Can you work these out from the model? Positions are in its coordinate system, mm. A direction names the side the tool comes from. Round coordinates to 2 decimals unless told otherwise and drop trailing zeros. Loops run counter-clockwise (first coordinate to the right, second up) from the corner with the lowest first, then second, coordinate; pieces in that order, holes last.
(1) Which directions (+Z, -Z, +X, -X, +Y, -Y) give clear straight access to the entire face, cutting with the end or side of a thin tool? Please do faces 1 (the face through (4.606, -3, 3)), 2 (the face through (-1, 150, 3)), 3 (the face through (4.606, 103, 3)).
(2) I want a section at C-C on x = 10.5. Write out the boundary of the cut face in (y, z).
(3) Will these pins go through, and if not, where does the flat tip stop? pin 1 Ø4 at (x, y) = (-20.39, 15) entering from +Z; pin 2 Ø2 at (x, y) = (-0.21, 80) entering from -Z.
(4) Thinking about a two-plate mould opening in X: for faces 4 (the face through (-5.394, -3, 3)), 5 (the face through (-0.48, 38.29, 3.04)), 6 (the face through (-16, 0, 3)), 7 (the face through (19.378, 26.735, 3.042)), which applies, released by +X, released by -X, zero draft, split by the parting line, or undercut?
(5) If I drill on line 1 along X through (y, z) = (65, 1.95); line 2 along Y through (x, z) = (-4, 4.35); line 3 along Y through (x, z) = (-18, 2.9), over which ranges is the centre line in solid material (lowest first)?
(6) I want a section at A-A on y = 40. Write out the boundary of the cut face in (x, z).
(7) I want a section at B-B on z = 4.65. Give the number of separate pieces and of enclosed holes in the cut face, plus the area to 3 significant figures.
from build123d import *

# Parameters (mm, degrees)
ESBO_O1_W                = 50
ESBO_O1_H                = 150
RESSALTO_EXTRUS_O1_DEPTH = 6
ESBO_O2_R                = 1.75
CORTE_EXTRUS_O1_DEPTH    = 6
ESBO_O3_W                = 10
ESBO_O3_H                = 6
RESSALTO_EXTRUS_O2_DEPTH = 6
ESBO_O4_W                = 10
ESBO_O4_H                = 6.295380903
CORTE_EXTRUS_O2_DEPTH    = 6
ESBO_O5_W                = 10
ESBO_O5_H                = 6
CORTE_EXTRUS_O3_DEPTH    = 6


with BuildPart() as part:
    # Esboço1 → Ressalto-extrusão1 (new body)
    with BuildSketch(Plane.XY):
        with Locations((-0.394283087, 75)):
            Rectangle(ESBO_O1_W, ESBO_O1_H)
    extrude(amount=RESSALTO_EXTRUS_O1_DEPTH)

    # Esboço2 → Corte-extrusão1 (cut)
    with BuildSketch(Plane.XY.offset(6)):
        with Locations((-20.394283087, 95)):
            Circle(ESBO_O2_R)
        with Locations((-20.394283087, 85)):
            Circle(ESBO_O2_R)
        with Locations((-20.394283087, 75)):
            Circle(ESBO_O2_R)
        with Locations((-20.394283087, 65)):
            Circle(ESBO_O2_R)
        with Locations((-20.394283087, 55)):
            Circle(ESBO_O2_R)
        with Locations((-20.394283087, 45)):
            Circle(ESBO_O2_R)
        with Locations((-20.394283087, 35)):
            Circle(ESBO_O2_R)
        with Locations((-20.394283087, 25)):
            Circle(ESBO_O2_R)
        with Locations((-20.394283087, 15)):
            Circle(ESBO_O2_R)
        with Locations((-20.394283087, 5)):
            Circle(ESBO_O2_R)
        with Locations((19.605716913, 95)):
            Circle(ESBO_O2_R)
        with Locations((19.605716913, 85)):
            Circle(ESBO_O2_R)
        with Locations((19.793101921, 75)):
            Circle(ESBO_O2_R)
        with Locations((19.793101921, 65)):
            Circle(ESBO_O2_R)
        with Locations((19.793101921, 55)):
            Circle(ESBO_O2_R)
        with Locations((19.605716913, 45)):
            Circle(ESBO_O2_R)
        with Locations((19.605716913, 35)):
            Circle(ESBO_O2_R)
        with Locations((19.605716913, 25)):
            Circle(ESBO_O2_R)
        with Locations((19.605716913, 15)):
            Circle(ESBO_O2_R)
        with Locations((19.605716913, 5)):
            Circle(ESBO_O2_R)
        with Locations((-0.052571078, 20)):
            Circle(ESBO_O2_R)
        with Locations((-0.210284313, 80)):
            Circle(ESBO_O2_R)
        with Locations((-0.105142156, 40)):
            Circle(ESBO_O2_R)
        with Locations((-0.157713235, 60)):
            Circle(ESBO_O2_R)
    extrude(amount=-CORTE_EXTRUS_O1_DEPTH, mode=Mode.SUBTRACT)

    # Esboço3 → Ressalto-extrusão2 (add)
    with BuildSketch(Plane(origin=(0, 0, 0), x_dir=(-1, 0, 0), z_dir=(0, -1, 0))):
        with Locations((0.394283087, -3)):
            Rectangle(ESBO_O3_W, ESBO_O3_H)
    extrude(amount=RESSALTO_EXTRUS_O2_DEPTH)

    # Esboço4 → Corte-extrusão2 (cut)
    with BuildSketch(Plane.XY.offset(6)):
        with Locations((-0.394283087, 103.147690452)):
            Rectangle(ESBO_O4_W, ESBO_O4_H)
    extrude(amount=-CORTE_EXTRUS_O2_DEPTH, mode=Mode.SUBTRACT)

    # Esboço5 → Corte-extrusão3 (cut)
    with BuildSketch(Plane.XY.offset(6)):
        with Locations((-0.394283087, 143.295380903)):
            Rectangle(ESBO_O5_W, ESBO_O5_H)
    extrude(amount=-CORTE_EXTRUS_O3_DEPTH, mode=Mode.SUBTRACT)


solid = part.part
Filled sheet:
1. face 1: +Z, -Z, +X, -Y
1. face 2: +Z, -Z, +X, -X, +Y
1. face 3: +Z, -Z
2. outline: (0, 0) - (150, 0) - (150, 6) - (0, 6) - close
3. pin 1: stops at z = 6
3. pin 2: passes through
4. face 4: released by -X
4. face 5: undercut
4. face 6: zero draft
4. face 7: undercut
5. line 1: x = -25.39 to -22.14, -18.64 to 18.04, 21.54 to 24.61
5. line 2: y = -6 to 100, 106.3 to 140.3, 146.3 to 150
5. line 3: y = 0 to 150
6. outline: (-25.39, 0) - (-1.86, 0) - (-1.86, 6) - (-25.39, 6) - close; (1.64, 0) - (24.61, 0) - (24.61, 6) - (1.64, 6) - close
7. separate pieces: 1
7. enclosed holes: 26
7. area: 7,210 mm2
